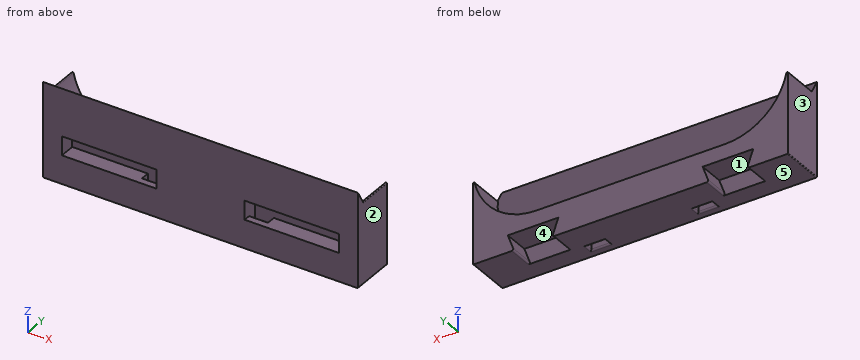
from build123d import *

# Parameters (mm, degrees)
SKETCH_1_W          = 200
SKETCH_1_H          = 60
EXTRUDE_1_DEPTH     = 28
CUT_EXTRUDE_1_DEPTH = 211.675105316
EXTRUDE_2_REACH     = 212.675
FILLET_1_R          = 0.5
CUT_EXTRUDE_START   = 12
CUT_EXTRUDE_2_DEPTH = 199.675105316
CUT_EXTRUDE_START_2 = 10
SKETCH_5_W          = 60
SKETCH_5_H          = 12
CUT_EXTRUDE_3_DEPTH = 221.675105316
SKETCH_6_W          = 12
SKETCH_6_H          = 5
CUT_EXTRUDE_4_DEPTH = 30
FILLET_2_R          = 1


with BuildPart() as part:
    # 草图1 → 凸台-拉伸1 (new body)
    with BuildSketch(Plane(origin=(0, 0, 0), x_dir=(1, 0, 0), z_dir=(0, 1, 0))):
        with Locations((100, -30)):
            Rectangle(SKETCH_1_W, SKETCH_1_H)
    extrude(amount=EXTRUDE_1_DEPTH)

    # 草图2 → 切除-拉伸1 (cut, through all)
    with BuildSketch(Plane(origin=(0, 0, 0), x_dir=(0, 0, -1), z_dir=(1, 0, 0))):
        Polygon((-60, 0), (-20, 23.094010768), (-20, 28), (-60, 28), align=None)
    extrude(amount=CUT_EXTRUDE_1_DEPTH, mode=Mode.SUBTRACT)

    # 凸台-拉伸2: up to this face of the body (flat: up to its plane)
    extrude_2_end = Plane(part.part.faces().sort_by_distance((100, 28, 10))[0])
    # 草图3 → 凸台-拉伸2 (add, up to the picked face)
    with BuildSketch(Plane(origin=(0, 0, 0), x_dir=(1, 0, 0), z_dir=(0, 1, 0)), mode=Mode.PRIVATE) as extrude_2_sk1:
        with BuildLine():
            Line((0, -60), (0, -20))
            Line((0, -20), (40, -20))
            ThreePointArc((40, -20), (11.715728753, -31.715728753), (0, -60))
        make_face()
    extrude_2_tool1 = split(extrude(extrude_2_sk1.sketch, amount=EXTRUDE_2_REACH, mode=Mode.PRIVATE), bisect_by=extrude_2_end, keep=Keep.BOTH, mode=Mode.PRIVATE)
    # 草图3 → 凸台-拉伸2 (add, up to the picked face)
    with BuildSketch(Plane(origin=(0, 0, 0), x_dir=(1, 0, 0), z_dir=(0, 1, 0)), mode=Mode.PRIVATE) as extrude_2_sk2:
        with BuildLine():
            Line((200, -20), (160, -20))
            ThreePointArc((160, -20), (188.284271247, -31.715728753), (200, -60))
            Line((200, -60), (200, -20))
        make_face()
    extrude_2_tool2 = split(extrude(extrude_2_sk2.sketch, amount=EXTRUDE_2_REACH, mode=Mode.PRIVATE), bisect_by=extrude_2_end, keep=Keep.BOTH, mode=Mode.PRIVATE)
    add(extrude_2_tool1.solids().sort_by(Axis((8.934718, 0, 28.934718), (0, 1, 0)))[0])
    add(extrude_2_tool2.solids().sort_by(Axis((191.065282, 0, 28.934718), (0, 1, 0)))[0])

    # 圆角1
    # the kernel refuses this fillet: 0.5 mm, written as the material it takes off along each edge
    with BuildSketch(Plane(origin=(200, -22.360679775, 60), x_dir=(-0.11111111111111022, 0, -0.9938079899999066), z_dir=(0, 1, 0))) as fillet_1_piece_1_section:
        with BuildLine():
            CenterArc((8.944444444, -0.496903995), FILLET_1_R, 96.379370208, 167.241259583)
            Line((8.888888889, -0.99380799), (0, 0))
            ThreePointArc((0, 0), (4.444444444, -0.2476804), (8.888888889, 0))
        make_face()
    fillet_1_piece_1 = extrude(amount=72.72135955, mode=Mode.PRIVATE)
    fillet_1_piece_1 = split(fillet_1_piece_1, bisect_by=Plane(origin=(199.731100006, 6.705360676, 48.385974626), z_dir=(0, 0.8660254037844379, 0.5000000000000012)), keep=Keep.TOP, mode=Mode.PRIVATE)
    add(fillet_1_piece_1, mode=Mode.SUBTRACT)
    with BuildSketch(Plane(origin=(0, -22.360679775, 60), x_dir=(0.11111111111111158, 0, -0.9938079899999065), z_dir=(0, 1, 0))) as fillet_1_piece_2_section:
        with BuildLine():
            CenterArc((8.944444444, 0.496903995), FILLET_1_R, 96.379370208, 167.241259583)
            Line((8.888888889, 0.99380799), (0, 0))
            ThreePointArc((0, 0), (4.444444444, 0.2476804), (8.888888889, 0))
        make_face()
    fillet_1_piece_2 = extrude(amount=72.72135955, mode=Mode.PRIVATE)
    fillet_1_piece_2 = split(fillet_1_piece_2, bisect_by=Plane(origin=(0.268899994, 6.705360676, 48.385974626), z_dir=(0, 0.8660254037844379, 0.5000000000000012)), keep=Keep.TOP, mode=Mode.PRIVATE)
    add(fillet_1_piece_2, mode=Mode.SUBTRACT)
    with BuildSketch(Plane(origin=(0, -1.25, 0), x_dir=(1, 0, 0), z_dir=(0, 1, 0))) as fillet_1_piece_3:
        with BuildLine():
            CenterArc((FILLET_1_R, -FILLET_1_R), FILLET_1_R, 90, 90)
            Line((0, -FILLET_1_R), (0, 0))
            Line((0, 0), (FILLET_1_R, 0))
        make_face()
    extrude(amount=30.5, mode=Mode.SUBTRACT)
    with BuildSketch(Plane(origin=(200, -1.25, 0), x_dir=(-1, 0, 0), z_dir=(0, 1, 0))) as fillet_1_piece_4:
        with BuildLine():
            CenterArc((FILLET_1_R, FILLET_1_R), FILLET_1_R, 180, 90)
            Line((0, FILLET_1_R), (0, 0))
            Line((0, 0), (FILLET_1_R, 0))
        make_face()
    extrude(amount=30.5, mode=Mode.SUBTRACT)

    # 草图4 → 切除-拉伸2 (cut, through all)
    with BuildSketch(Plane(origin=(0, 0, 0), x_dir=(1, 0, 0), z_dir=(0, 1, 0)).offset(CUT_EXTRUDE_START)):
        Polygon((26, 0), (22.105518493, -10.7), (54.194481507, -10.7), (50.3, 0), align=None)
        Polygon((145.805518493, -10.7), (149.7, 0), (174, 0), (177.894481507, -10.7), align=None)
    extrude(amount=CUT_EXTRUDE_2_DEPTH, mode=Mode.SUBTRACT)

    # 草图5 → 切除-拉伸3 (cut, through all)
    with BuildSketch(Plane(origin=(0, 0, 0), x_dir=(1, 0, 0), z_dir=(0, 1, 0)).offset(CUT_EXTRUDE_START_2)):
        with Locations((42, -24)):
            Rectangle(SKETCH_5_W, SKETCH_5_H)
        with Locations((158, -24)):
            Rectangle(SKETCH_5_W, SKETCH_5_H)
    extrude(amount=-CUT_EXTRUDE_3_DEPTH, mode=Mode.SUBTRACT)

    # 草图6 → 切除-拉伸4 (cut)
    with BuildSketch(Plane.XY):
        with Locations((66, 7.5)):
            Rectangle(SKETCH_6_W, SKETCH_6_H)
        with Locations((134, 7.5)):
            Rectangle(SKETCH_6_W, SKETCH_6_H)
    extrude(amount=CUT_EXTRUDE_4_DEPTH, mode=Mode.SUBTRACT)

    # 圆角2
    fillet_2_edges = [part.edges().sort_by_distance(p)[0] for p in [
        (50.3, 20, 0),
        (26, 20, 0),
        (174, 20, 0),
        (149.7, 20, 0),
        (66, 5, 0),
        (66, 10, 0),
        (60, 7.5, 0),
        (72, 7.5, 0),
        (66, 5, 18),
        (134, 10, 0),
        (134, 5, 0),
        (128, 7.5, 0),
        (140, 7.5, 0),
        (134, 5, 18),
    ]]
    fillet(fillet_2_edges, radius=FILLET_2_R)


solid = part.part
Verification items for the finished model (mm, model axes). Face numbers are marked on the shaded views. A direction names the side the tool comes from. Give positions to 0.01 mm unless a question says otherwise; leave off trailing zeros. Loops run counter-clockwise (first coordinate to the right, second up) from the corner with the lowest first, then second, coordinate; pieces in that order, holes last.
1) Depth check by flat-ended pin: pin 1 Ø2.5 at (x, y) = (111.5, 25.5) entering from +Z; pin 2 Ø1 at (x, z) = (111, 20.5) entering from -Y; pin 3 Ø4 at (x, y) = (126.5, 21) entering from +Z; pin 4 Ø6 at (x, z) = (135, 26) entering from -Y. Enter the tip coordinate at first touch or a pass-through.
2) Thickness scan on line 1 along X through (y, z) = (9.5, 26.5); line 2 along Z through (x, y) = (157.5, 25.25); line 3 along X through (y, z) = (12.25, 5.5). Record the ranges inside material, lowest first.
3) Set-up check for the marked faces 1 and 2: record each of +Z, -Z, +X, -X, +Y, -Y from which the full face is reachable in a straight line by a thin tool's end or side.
4) Draft check along X on the marked faces 3, 4 and 5. Enter one of: pulls with the +X half, pulls with the -X half, needs draft (parallel to the pull), parting line crosses it, or undercut.
5) Sectioned sample at A-A, the plane x = 57. Enter the section's corners in (y, z), then the cut area to 3 significant figures.
6) Sectioned sample at B-B, the plane z = 5.5. Enter the section's corners in (x, y), then the cut area to 3 significant figures.
7) Sectioned sample at D-D, the plane z = 38. Enter the section's corners in (x, y), then the cut area to 3 significant figures.
8) Sectioned sample at C-C, the plane y = 16. Enter the section's corners in (x, z).
Answers:
1. pin 1: stops at z = 20
1. pin 2: stops at y = 0
1. pin 3: stops at z = 27.09
1. pin 4: stops at y = 10
2. line 1: x = 0 to 12, 72 to 128, 188 to 200
2. line 2: z = 10.7 to 20
2. line 3: x = 0 to 24, 52.3 to 147.7, 176 to 200
3. face 1: +Y
3. face 2: +Z, -Z, +X, +Y, -Y
4. face 3: pulls with the -X half
4. face 4: undercut
4. face 5: needs draft
5. outline: (0, 0) - (28, 0) - (28, 20) - (23.09, 20) - (0, 60) - (0, 30) - (10, 30) - (10, 18) - (0, 18) - close
5. area: 902 mm2
6. outline: (0, 0) - (200, 0) - (200, 28) - (176, 28) - (176, 12) - (147.7, 12) - (147.7, 28) - (52.3, 28) - (52.3, 12) - (24, 12) - (24, 28) - (0, 28) - close; hole (60, 5) - (72, 5) - (72, 10) - (60, 10) - close; hole (128, 5) - (140, 5) - (140, 10) - (128, 10) - close
6. area: 4,570 mm2
7. outline: (0, 0) - (200, 0) - (200, 28) - (193.41, 28) - (193.41, 12.7) - (6.59, 12.7) - (6.59, 28) - (0, 28) - close
7. area: 2,740 mm2
8. outline: (0, 0.5) arc R0.5 ccw to (0.5, 0) - (24.57, 0) arc R1 ccw to (25.51, 1.34) - (22.11, 10.7) - (54.19, 10.7) - (50.79, 1.34) arc R1 ccw to (51.73, 0) - (148.27, 0) arc R1 ccw to (149.21, 1.34) - (145.81, 10.7) - (177.89, 10.7) - (174.49, 1.34) arc R1 ccw to (175.43, 0) - (199.5, 0) arc R0.5 ccw to (200, 0.5) - (200, 51.06) arc R0.5 ccw to (199.01, 51.17) arc R40 cw to (188.84, 32.29) - (11.16, 32.29) arc R40 cw to (0.99, 51.17) arc R0.5 ccw to (0, 51.06) - close
